The listing builds one solid part. Answer for the finished solid, in the listing's coordinates (mm). Give positions to 0.01 mm unless a question says otherwise; leave off trailing zeros. Loops run counter-clockwise (first coordinate to the right, second up) from the corner with the lowest first, then second, coordinate; pieces in that order, holes last.
Item 1: Consider line 1 along Y through (x, z) = (0, -119.5); line 2 along X through (y, z) = (-0.5, 118); line 3 along Y through (x, z) = (-1, 100). Determine where each line is inside the solid, lowest interval first.
Item 2: Section A-A, the plane z = -21 is taken. Give the vertices of the cut face in (x, y).
Item 3: Each of these flat-tipped pins is pushed along its axis until it touches: pin 1 Ø4.5 at (x, y) = (0, 0) entering from -Z; pin 2 Ø5 at (x, y) = (0, 0) entering from -Z. Where does it stop, or does it pass through?
from build123d import *

# Parameters (mm, degrees)
BOSS_EXTRUDE1_DEPTH               = 129
F_1_4_28_TAPPED_HOLE1_D           = 5.4102
F_1_4_28_TAPPED_HOLE1_DEPTH       = 15.24
F_1_4_28_TAPPED_HOLE1_CSINK_D     = 7.62
F_1_4_28_TAPPED_HOLE1_CSINK_ANGLE = 90
F_1_4_28_TAPPED_HOLE1_TIP         = 1.625388061
F_1_4_28_TAPPED_HOLE2_D           = 5.4102
F_1_4_28_TAPPED_HOLE2_DEPTH       = 17.2339
F_1_4_28_TAPPED_HOLE2_CSINK_D     = 7.62
F_1_4_28_TAPPED_HOLE2_CSINK_ANGLE = 90
F_1_4_28_TAPPED_HOLE2_TIP         = 1.625388061


with BuildPart() as part:
    # Sketch3 → Boss-Extrude1 (new, symmetric)
    with BuildSketch(Plane.XY):
        Polygon((0, 5.499261314), (4.7625, 2.749630657), (4.7625, -2.749630657), (0, -5.499261314), (-4.7625, -2.749630657), (-4.7625, 2.749630657), align=None)
    extrude(amount=BOSS_EXTRUDE1_DEPTH, both=True)

    # 1/4-28 Tapped Hole1
    with Locations(Plane.XY.offset(129)):
        with Locations((0, 0)):
            CounterSinkHole(F_1_4_28_TAPPED_HOLE1_D / 2, F_1_4_28_TAPPED_HOLE1_CSINK_D / 2, depth=F_1_4_28_TAPPED_HOLE1_DEPTH, counter_sink_angle=F_1_4_28_TAPPED_HOLE1_CSINK_ANGLE)
            with Locations((0, 0, -(F_1_4_28_TAPPED_HOLE1_DEPTH + F_1_4_28_TAPPED_HOLE1_TIP / 2))):  # 118° drill point
                Cone(0, F_1_4_28_TAPPED_HOLE1_D / 2, F_1_4_28_TAPPED_HOLE1_TIP, mode=Mode.SUBTRACT)

    # 1/4-28 Tapped Hole2
    with Locations(Plane(origin=(0, 0, -129), x_dir=(-1, 0, 0), z_dir=(0, 0, -1))):
        with Locations((0, 0)):
            CounterSinkHole(F_1_4_28_TAPPED_HOLE2_D / 2, F_1_4_28_TAPPED_HOLE2_CSINK_D / 2, depth=F_1_4_28_TAPPED_HOLE2_DEPTH, counter_sink_angle=F_1_4_28_TAPPED_HOLE2_CSINK_ANGLE)
            with Locations((0, 0, -(F_1_4_28_TAPPED_HOLE2_DEPTH + F_1_4_28_TAPPED_HOLE2_TIP / 2))):  # 118° drill point
                Cone(0, F_1_4_28_TAPPED_HOLE2_D / 2, F_1_4_28_TAPPED_HOLE2_TIP, mode=Mode.SUBTRACT)


solid = part.part
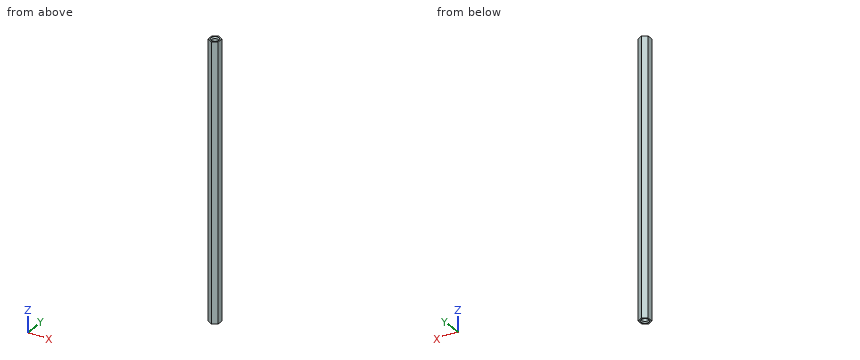
Worked answers:
1. line 1: y = -5.5 to -2.71, 2.71 to 5.5
1. line 2: x = -4.76 to -2.66, 2.66 to 4.76
1. line 3: y = -4.92 to 4.92
2. outline: (-4.76, -2.75) - (0, -5.5) - (4.76, -2.75) - (4.76, 2.75) - (0, 5.5) - (-4.76, 2.75) - close
3. pin 1: stops at z = -111.49
3. pin 2: stops at z = -111.64
